The model under review builds one solid part; all positions refer to its coordinate system, in mm. A direction names the side the tool comes from. Round coordinates to 2 decimals unless told otherwise and drop trailing zeros. Loops run counter-clockwise (first coordinate to the right, second up) from the corner with the lowest first, then second, coordinate; pieces in that order, holes last. Notation, with made-up numbers: (-1, 4.5) -> (36, 4.5) arc R19 cw to (36, 14.5) -> close; hole circle Ø11 at (-26.5, 3.25). An arc over 180 degrees is marked (long way). Use CSV: the item, a comma, the result in double quotes. Start each with the question number.
```python
from build123d import *

# Parameters (mm, degrees)
SKETCH1_W           = 85
SKETCH1_H           = 50
BOSS_EXTRUDE1_DEPTH = 6
BOSS_EXTRUDE2_DEPTH = 4
SKETCH4_R           = 2.5
CUT_EXTRUDE2_DEPTH  = 11
SKETCH5_W           = 55
SKETCH5_H           = 35
BOSS_EXTRUDE3_DEPTH = 16.7
FILLET1_R           = 5
SKETCH6_R           = 1.74
CUT_EXTRUDE3_DEPTH  = 10
SKETCH7_W           = 25
SKETCH7_H           = 35
CUT_EXTRUDE4_DEPTH  = 12.7
FILLET3_R           = 4
FILLET4_R           = 4
FILLET5_R           = 4
CHAMFER1_SIZE       = 0.25


with BuildPart() as part:
    # Sketch1 → Boss-Extrude1 (new body)
    with BuildSketch(Plane(origin=(0, 0, 0), x_dir=(1, 0, 0), z_dir=(0, 1, 0))):
        with Locations((42.5, 25)):
            Rectangle(SKETCH1_W, SKETCH1_H)
    extrude(amount=BOSS_EXTRUDE1_DEPTH)

    # Sketch2 → Boss-Extrude2 (add)
    with BuildSketch(Plane(origin=(0, 6, 0), x_dir=(1, 0, 0), z_dir=(0, 1, 0))):
        Polygon((0, 0), (0, 50), (24.574331447, 50), (24.574331447, 35), (9.574331447, 35), (9.574331447, 0), align=None)
    extrude(amount=BOSS_EXTRUDE2_DEPTH)

    # Sketch4 → Cut-Extrude2 (cut)
    with BuildSketch(Plane(origin=(0, 10, 0), x_dir=(1, 0, 0), z_dir=(0, 1, 0))):
        with Locations((18.574331447, 42.5)):
            Circle(SKETCH4_R)
        with Locations((8.574331447, 42.5)):
            Circle(SKETCH4_R)
    extrude(amount=-CUT_EXTRUDE2_DEPTH, mode=Mode.SUBTRACT)

    # Sketch5 → Boss-Extrude3 (add)
    with BuildSketch(Plane(origin=(0, 6, 0), x_dir=(1, 0, 0), z_dir=(0, 1, 0))):
        with Locations((37.074331447, 17.5)):
            Rectangle(SKETCH5_W, SKETCH5_H)
    extrude(amount=BOSS_EXTRUDE3_DEPTH)

    # Fillet1
    fillet1_edges = [part.edges().sort_by_distance(p)[0] for p in [
        (0, 5, -50),
        (85, 3, -50),
        (85, 3, 0),
        (0, 5, 0),
    ]]
    fillet(fillet1_edges, radius=FILLET1_R)

    # Sketch6 → Cut-Extrude3 (cut)
    with BuildSketch(Plane(origin=(0, 22.7, 0), x_dir=(1, 0, 0), z_dir=(0, 1, 0))):
        with Locations((60.324331447, 26.5)):
            Circle(SKETCH6_R)
        with Locations((60.324331447, 8.5)):
            Circle(SKETCH6_R)
    extrude(amount=-CUT_EXTRUDE3_DEPTH, mode=Mode.SUBTRACT)

    # Sketch7 → Cut-Extrude4 (cut)
    with BuildSketch(Plane(origin=(0, 22.7, 0), x_dir=(1, 0, 0), z_dir=(0, 1, 0))):
        with Locations((22.074331447, 17.5)):
            Rectangle(SKETCH7_W, SKETCH7_H)
    extrude(amount=-CUT_EXTRUDE4_DEPTH, mode=Mode.SUBTRACT)

    # Fillet3
    fillet3_edges = [part.edges().sort_by_distance(p)[0] for p in [
        (34.574331447, 16.35, 0),
        (34.574331447, 16.35, -35),
        (64.574331447, 14.35, -35),
        (64.574331447, 14.35, 0),
    ]]
    fillet(fillet3_edges, radius=FILLET3_R)

    # Fillet4
    fillet4_edges = [part.edges().sort_by_distance(p)[0] for p in [
        (24.574331447, 8, -35),
    ]]
    fillet(fillet4_edges, radius=FILLET4_R)

    # Fillet5
    fillet5_edges = [part.edges().sort_by_distance(p)[0] for p in [
        (24.574331447, 8, -50),
    ]]
    fillet(fillet5_edges, radius=FILLET5_R)

    # Chamfer1
    chamfer1_edges = [part.edges().sort_by_distance(p)[0] for p in [
        (16.074331447, 10, -42.5),
        (6.074331447, 10, -42.5),
        (58.584331447, 22.7, -26.5),
        (58.584331447, 22.7, -8.5),
    ]]
    chamfer(chamfer1_edges, length=CHAMFER1_SIZE)


solid = part.part
```
1. The part is to be moulded in two halves that separate along X. For faces 1 (the face through (20.884, 4.943, -41.542)), 2 (the face through (35.78, 16.26, -1.14)), 3 (the face through (64.574, 14, -17)), 4 (the face through (42, 9, 0)), say which applies: pulls with the +X half, pulls with the -X half, needs draft (parallel to the pull), parting line crosses it, or undercut.
2. Take a section at C-C, the plane z = -26.5. Give the boundary of the cut face in (x, y), then the cut area to 3 significant figures.
3. For line 1 along X through (y, z) = (6.75, -42.5); line 2 along X through (y, z) = (20.25, -26.5); line 3 along Z through (x, y) = (60, 14.5), list the stretches that pass through material, from the lowest coordinate up. Write a range as from..to.
4. For faces 5 (the face through (2, 5, -1)), 6 (the face through (34.574, 16, -17)), 7 (the face through (60, 12.7, -27)), 8 (the face through (1, 5, -48)), 9 (the face through (24.574, 8, -43)), list the 3-axis set-ups (+Z, -Z, +X, -X, +Y, -Y) from which the entire face can be reached by the end or side of a thin tool; tool diameter is ignored.
5. Clearance check with flat-ended pins moving along their axes: P1, Ø5, axis at x = 47, y = 8, coming from the -Z side; P2, Ø1.5, axis at y = 16.5, z = -6, coming from the -X side; P3, Ø3, axis at x = 60.32, z = -26.5, coming from the +Y side; P4, Ø6.5, axis at x = 18.57, z = -42.5, coming from the +Y side. State where each tip first meets the part, or that it passes through.
6. Take a section at B-B, the plane y = 8.5. Give the boundary of the cut face in (x, z).
7. Take a section at D-D, the plane x = 50. Give the boundary of the cut face in (y, z), then the cut area to 4 significant figures.
8. Take a section at A-A, the plane z = -42.5. Give the boundary of the cut face in (x, y).
Results:
1,face 1,"undercut"
1,face 2,"pulls with the -X half"
1,face 3,"pulls with the +X half"
1,face 4,"needs draft"
2,outline,"(0, 0) -> (85, 0) -> (85, 6) -> (64.57, 6) -> (64.57, 22.7) -> (62.31, 22.7) -> (62.06, 22.45) -> (62.06, 12.7) -> (58.58, 12.7) -> (58.58, 22.45) -> (58.33, 22.7) -> (34.57, 22.7) -> (34.57, 10) -> (0, 10) -> close"
2,area,"1,110 mm²"
3,line 1,"0..6.07, 11.07..16.07, 21.07..24.57"
3,line 2,"34.57..58.58, 62.06..64.57"
3,line 3,"-35..-28.21, -24.79..-10.21, -6.79..0"
4,face 5,"+Z, -X, +Y, -Y"
4,face 6,"+Z, -Z, -X, +Y"
4,face 7,"+Y"
4,face 8,"-Z, -X, +Y, -Y"
4,face 9,"-Z, +X, +Y"
5,P1,"z = -50"
5,P2,"x = 34.57"
5,P3,"y = 12.7"
5,P4,"y = 10"
6,outline,"(0, -45) arc R5 ccw to (5, -50) -> (20.57, -50) arc R4 ccw to (24.57, -46) -> (24.57, -39) arc R4 cw to (28.57, -35) -> (60.57, -35) arc R4 ccw to (64.57, -31) -> (64.57, -4) arc R4 ccw to (60.57, 0) -> (5, 0) arc R5 ccw to (0, -5) -> close; hole circle Ø5 at (8.57, -42.5); hole circle Ø5 at (18.57, -42.5)"
7,outline,"(0, -50) -> (6, -50) -> (6, -35) -> (22.7, -35) -> (22.7, 0) -> (0, 0) -> close"
7,area,"884.5 mm²"
8,outline,"(0, 0) -> (6.07, 0) -> (6.07, 9.75) -> (5.82, 10) -> (0, 10) -> close; (11.07, 0) -> (16.07, 0) -> (16.07, 9.75) -> (15.82, 10) -> (11.32, 10) -> (11.07, 9.75) -> close; (21.07, 0) -> (85, 0) -> (85, 6) -> (24.57, 6) -> (24.57, 10) -> (21.32, 10) -> (21.07, 9.75) -> close"
